```python
from build123d import *

# Parameters (mm, degrees)
BOSS_EXTRUDE1_DEPTH    = 18
CUT_EXTRUDE1_DEPTH     = 10
CHAMFER1_SIZE          = 3
CUT_EXTRUDE5_START     = -15.5
CUT_EXTRUDE5_DEPTH     = 15.5
CUT_EXTRUDE6_DEPTH     = 4.5
SKETCH3_6_R            = 2.25
CUT_EXTRUDE8_DEPTH     = 7
CUT_EXTRUDE9_START     = -2.5
CUT_EXTRUDE9_OUTLINE_W = 18.5
CUT_EXTRUDE9_OUTLINE_H = 12
CUT_EXTRUDE9_OUTLINE_R = 6
CUT_EXTRUDE9_DEPTH     = 2.5
CUT_EXTRUDE17_START    = -13
SKETCH8_R              = 4
CUT_EXTRUDE17_DEPTH    = 13
CHAMFER2_SIZE          = 0.8
SKETCH10_R             = 7
SKETCH10_R_2           = 6
CUT_EXTRUDE19_DEPTH    = 1.2


# Read off the part's stored shape, not the designer's step: Cut-Extrude9
with BuildPart() as part:
    # Sketch1 → Boss-Extrude1 (new body)
    with BuildSketch(Plane(origin=(0, 0, 0), x_dir=(1, 0, 0), z_dir=(0, 1, 0))):
        with BuildLine():
            Line((-67.5, -77.5), (67.5, -77.5))
            ThreePointArc((67.5, -77.5), (74.571067812, -74.571067812), (77.5, -67.5))
            Line((77.5, -67.5), (77.5, 67.5))
            ThreePointArc((77.5, 67.5), (74.571067812, 74.571067812), (67.5, 77.5))
            Line((67.5, 77.5), (-67.5, 77.5))
            ThreePointArc((-67.5, 77.5), (-74.571067812, 74.571067812), (-77.5, 67.5))
            Line((-77.5, 67.5), (-77.5, -67.5))
            ThreePointArc((-77.5, -67.5), (-74.571067812, -74.571067812), (-67.5, -77.5))
        make_face()
    extrude(amount=BOSS_EXTRUDE1_DEPTH)

    # Sketch2 → Cut-Extrude1 (cut)
    with BuildSketch(Plane(origin=(0, 0, 0), x_dir=(1, 0, 0), z_dir=(0, 1, 0))):
        with BuildLine():
            Line((77.5, -67.5), (77.5, 67.5))
            ThreePointArc((77.5, 67.5), (74.571067812, 74.571067812), (67.5, 77.5))
            Line((67.5, 77.5), (-67.5, 77.5))
            ThreePointArc((-67.5, 77.5), (-74.571067812, 74.571067812), (-77.5, 67.5))
            Line((-77.5, 67.5), (-77.5, -67.5))
            ThreePointArc((-77.5, -67.5), (-74.571067812, -74.571067812), (-67.5, -77.5))
            Line((-67.5, -77.5), (67.5, -77.5))
            ThreePointArc((67.5, -77.5), (74.571067812, -74.571067812), (77.5, -67.5))
        make_face()
        with BuildLine():
            Line((-74.5, 67.5), (-74.5, -67.5))
            ThreePointArc((-74.5, -67.5), (-72.449747468, -72.449747468), (-67.5, -74.5))
            Line((-67.5, -74.5), (67.5, -74.5))
            ThreePointArc((67.5, -74.5), (72.449747468, -72.449747468), (74.5, -67.5))
            Line((74.5, -67.5), (74.5, 67.5))
            ThreePointArc((74.5, 67.5), (72.449747468, 72.449747468), (67.5, 74.5))
            Line((67.5, 74.5), (-67.5, 74.5))
            ThreePointArc((-67.5, 74.5), (-72.449747468, 72.449747468), (-74.5, 67.5))
        make_face(mode=Mode.SUBTRACT)
    extrude(amount=CUT_EXTRUDE1_DEPTH, mode=Mode.SUBTRACT)

    # Chamfer1
    chamfer1_edges = [part.edges().sort_by_distance(p)[0] for p in [
        (-72.449747468, 10, -72.449747468),
        (-74.5, 10, 0),
        (-72.449747468, 10, 72.449747468),
        (0, 10, 74.5),
        (72.449747468, 10, 72.449747468),
        (74.5, 10, 0),
        (72.449747468, 10, -72.449747468),
        (0, 10, -74.5),
    ]]
    chamfer(chamfer1_edges, length=CHAMFER1_SIZE - 0.0001)  # a hair under: the kernel refuses the full size

    # Sketch3 → Cut-Extrude5 (cut)
    with BuildSketch(Plane(origin=(0, 18, 0), x_dir=(1, 0, 0), z_dir=(0, 1, 0)).offset(CUT_EXTRUDE5_START)):
        with BuildLine():
            Line((67.5, 58.5), (70.5, 58.5))
            Line((70.5, 58.5), (70.5, -58.584654437))
            Line((70.5, -58.584654437), (66.268491377, -58.584654437))
            ThreePointArc((66.268491377, -58.584654437), (60.714590005, -61.58745307), (58.5, -67.5))
            Line((58.5, -67.5), (58.5, -70.5))
            Line((58.5, -70.5), (-58.584654437, -70.5))
            Line((-58.584654437, -70.5), (-58.584654437, -66.268491377))
            ThreePointArc((-58.584654437, -66.268491377), (-61.58745307, -60.714590005), (-67.5, -58.5))
            Line((-67.5, -58.5), (-70.5, -58.5))
            Line((-70.5, -58.5), (-70.5, 58.584654437))
            Line((-70.5, 58.584654437), (-66.268491377, 58.584654437))
            ThreePointArc((-66.268491377, 58.584654437), (-60.714590005, 61.58745307), (-58.5, 67.5))
            Line((-58.5, 67.5), (-58.5, 70.5))
            Line((-58.5, 70.5), (58.584654437, 70.5))
            Line((58.584654437, 70.5), (58.584654437, 66.268491377))
            ThreePointArc((58.584654437, 66.268491377), (61.58745307, 60.714590005), (67.5, 58.5))
        make_face()
    extrude(amount=CUT_EXTRUDE5_DEPTH, mode=Mode.SUBTRACT)

    # Sketch3<5> → Cut-Extrude6 (cut)
    with BuildSketch(Plane(origin=(0, 18, 0), x_dir=(1, 0, 0), z_dir=(0, 1, 0))):
        with BuildLine():
            Line((75.5, -63.542327218), (75.5, 63.5))
            Line((75.5, 63.5), (67.5, 63.5))
            ThreePointArc((67.5, 63.5), (64.884801062, 64.473329467), (63.542327218, 66.919632742))
            Line((63.542327218, 66.919632742), (63.542327218, 75.5))
            Line((63.542327218, 75.5), (-63.5, 75.5))
            Line((-63.5, 75.5), (-63.5, 67.5))
            ThreePointArc((-63.5, 67.5), (-64.473329467, 64.884801062), (-66.919632742, 63.542327218))
            Line((-66.919632742, 63.542327218), (-75.5, 63.542327218))
            Line((-75.5, 63.542327218), (-75.5, -63.5))
            Line((-75.5, -63.5), (-67.5, -63.5))
            ThreePointArc((-67.5, -63.5), (-64.884801062, -64.473329467), (-63.542327218, -66.919632742))
            Line((-63.542327218, -66.919632742), (-63.542327218, -75.5))
            Line((-63.542327218, -75.5), (63.5, -75.5))
            Line((63.5, -75.5), (63.5, -67.5))
            ThreePointArc((63.5, -67.5), (64.473329467, -64.884801062), (66.919632742, -63.542327218))
            Line((66.919632742, -63.542327218), (75.5, -63.542327218))
        make_face()
        with BuildLine():
            Line((-67.5, -59.5), (-71.5, -59.5))
            Line((-71.5, -59.5), (-71.5, 59.584654437))
            Line((-71.5, 59.584654437), (-66.339265485, 59.584654437))
            ThreePointArc((-66.339265485, 59.584654437), (-61.446658934, 62.269602124), (-59.5, 67.5))
            Line((-59.5, 67.5), (-59.5, 71.5))
            Line((-59.5, 71.5), (59.584654437, 71.5))
            Line((59.584654437, 71.5), (59.584654437, 66.339265485))
            ThreePointArc((59.584654437, 66.339265485), (62.269602124, 61.446658934), (67.5, 59.5))
            Line((67.5, 59.5), (71.5, 59.5))
            Line((71.5, 59.5), (71.5, -59.584654437))
            Line((71.5, -59.584654437), (66.339265485, -59.584654437))
            ThreePointArc((66.339265485, -59.584654437), (61.446658934, -62.269602124), (59.5, -67.5))
            Line((59.5, -67.5), (59.5, -71.5))
            Line((59.5, -71.5), (-59.584654437, -71.5))
            Line((-59.584654437, -71.5), (-59.584654437, -66.339265485))
            ThreePointArc((-59.584654437, -66.339265485), (-62.269602124, -61.446658934), (-67.5, -59.5))
        make_face(mode=Mode.SUBTRACT)
    extrude(amount=-CUT_EXTRUDE6_DEPTH, mode=Mode.SUBTRACT)

    # Sketch3<6> → Cut-Extrude8 (cut)
    with BuildSketch(Plane(origin=(0, 18, 0), x_dir=(1, 0, 0), z_dir=(0, 1, 0))):
        with Locations(Location((-67.5, -67.5, 0), (0, 0, 270))):
            Circle(SKETCH3_6_R)
        with Locations(Location((-67.5, 67.5, 0), (0, 0, 270))):
            Circle(SKETCH3_6_R)
        with Locations(Location((67.5, 67.5, 0), (0, 0, 270))):
            Circle(SKETCH3_6_R)
        with Locations(Location((67.5, -67.5, 0), (0, 0, 270))):
            Circle(SKETCH3_6_R)
    extrude(amount=-CUT_EXTRUDE8_DEPTH, mode=Mode.SUBTRACT)

    # Cut-Extrude9 outline → Cut-Extrude9 (cut)
    with BuildSketch(Plane(origin=(0, 2.5, 0), x_dir=(1, 0, 0), z_dir=(0, 1, 0)).offset(CUT_EXTRUDE9_START)):
        with Locations((20.5, -40.5)):
            Rectangle(CUT_EXTRUDE9_OUTLINE_W, CUT_EXTRUDE9_OUTLINE_H)
        with Locations((-24.5, -40.5)):
            Circle(CUT_EXTRUDE9_OUTLINE_R)
        with Locations((-4.5, -40.5)):
            Circle(CUT_EXTRUDE9_OUTLINE_R)
        with Locations((-44.5, -40.5)):
            Circle(CUT_EXTRUDE9_OUTLINE_R)
    extrude(amount=CUT_EXTRUDE9_DEPTH, mode=Mode.SUBTRACT)

    # Sketch8 → Cut-Extrude17 (cut)
    with BuildSketch(Plane.XZ.offset(CUT_EXTRUDE17_START)):
        with Locations(Location((67.5, 67.5, 0), (0, 0, 270))):
            Circle(SKETCH8_R)
        with Locations(Location((67.5, -67.5, 0), (0, 0, 270))):
            Circle(SKETCH8_R)
        with Locations(Location((-67.5, -67.5, 0), (0, 0, 270))):
            Circle(SKETCH8_R)
        with Locations(Location((-67.5, 67.5, 0), (0, 0, 270))):
            Circle(SKETCH8_R)
    extrude(amount=CUT_EXTRUDE17_DEPTH, mode=Mode.SUBTRACT)

    # Chamfer2
    chamfer2_edges = [part.edges().sort_by_distance(p)[0] for p in [
        (-67.5, 13, 71.5),
        (-67.5, 13, 65.25),
        (-67.5, 13, -63.5),
        (-67.5, 13, -69.75),
        (67.5, 13, -63.5),
        (67.5, 13, -69.75),
        (67.5, 13, 71.5),
        (67.5, 13, 65.25),
    ]]
    chamfer(chamfer2_edges, length=CHAMFER2_SIZE)

    # Sketch10 → Cut-Extrude19 (cut)
    with BuildSketch(Plane.XZ):
        with Locations(Location((-4.5, 40.5, 0), (0, 0, 270))):
            Circle(SKETCH10_R)
        with Locations(Location((-4.5, 40.5, 0), (0, 0, 90))):
            Circle(SKETCH10_R_2, mode=Mode.SUBTRACT)
    extrude(amount=-CUT_EXTRUDE19_DEPTH, mode=Mode.SUBTRACT)


solid = part.part
```
For this review, take the finished solid that the model builds, in its own axes (mm). A direction names the side the tool comes from. Round coordinates to 2 decimals unless told otherwise and drop trailing zeros. Use one line per item in the form item = value.
1) Clearance check with flat-ended pins moving along their axes: pin 1 (3 mm diameter, centred on x = -52, y = 3.5, fed in from -Z); pin 2 (10 mm diameter, centred on x = -51.5, z = 62, fed in from +Y); pin 3 (2 mm diameter, centred on x = 70, y = 17, fed in from -Z). State where each tip first meets the part, or that it passes through.
Found:
pin_1 = -74.5
pin_2 = 2.5
pin_3 = -77.39
2) Tool access review of faces 1 (the flat face through (-75.5, 16, -1)), 2 (the flat face through (-1, 1.2, 35)), 3 (the cylindrical face through (65.304, 15.929, 67.012)): name each direction out of +Z, -Z, +X, -X, +Y, -Y from which nothing blocks a thin tool from reaching the whole face with its end or side.
Found:
face_1 = +Y
face_2 = -Y
face_3 = +Y, -Y
3) Mouldability with a two-part tool opening along Z and no side actions: class faces 4 (the cylindrical face through (72.5, 3.5, -72.4)), 5 (the cylindrical face through (-71.049, 6.185, -69.346)), 6 (the flat face through (-1, 3, 74.5)), 7 (the cylindrical face through (61.52, 10.142, -60.774)) as +Z half, -Z half, draft (parallel to the pull), parting line (faces both ways), or undercut.
Found:
face_4 = -Z half
face_5 = undercut
face_6 = +Z half
face_7 = undercut
4) Take a section at D-D, the plane z = 40.5. Count the separate pieces of the cut face and the enclosed holes in it, and give its area (3 significant figures).
Found:
separate_pieces = 5
enclosed_holes = 0
area = 379 mm2
5) To check wall thickness, follow L1, parallel to X at y = 17.1, z = -67.5; L2, parallel to X at y = 5, z = -67.5; L3, parallel to X at y = 15.5, z = 2. State the ranges of each line that lie inside material, in increasing order. Write a range as from..to.
Found:
L1 = -77.5..-69.75, -65.25..-63.5, -59.5..-58.5, 58.58..59.58, 63.54..65.25, 69.75..77.5
L2 = -74.5..-71.5, -63.5..-58.5, 58.58..63.5, 71.5..74.5
L3 = -77.5..-75.5, -71.5..-70.5, 70.5..71.5, 75.5..77.5
